Design review of the part built by this model. Coordinates are the model's own, in mm. Face numbers are marked on the shaded views. A direction names the side the tool comes from. Give positions to 0.01 mm unless a question says otherwise; leave off trailing zeros. Order: outer loops, then holes, each group sorted by start corner. A loop starts at its lowest first (then second) coordinate and runs counter-clockwise, first axis right, second up. Notation, with made-up numbers: (65.5, 33.5) -> (109.5, 33.5) arc R25 cw to (109.5, 45.5) -> close; hole circle Ø3 at (-8, 53). An arc over 180 degrees is marked (long way). One line per item, written item: value. Start each with the question number.
1) The part is to be moulded in two halves that separate along X. For the marked faces 1, 2 and 3, say which applies: released by +X, released by -X, zero draft, split by the parting line, or undercut.
2) Consider section C-C (y = 0). State the section outline as (x, z) points.
3) Wall thickness on line 1 along Y through (x, z) = (39, 2.5); line 2 along Y through (x, z) = (-21, 2.95); line 3 along Z through (x, y) = (-27, -4.5): over which ranges is each line inside the solid? List them lowest first. Write a range as from..to.
4) For pin 1 (7 mm diameter, centred on x = -21, y = 0, fed in from -Z), flat-tipped, find the tip position at first contact; note if it passes through.
5) Consider section A-A (z = 2). State the section outline as (x, y) points, plus the area to 3 significant figures.
6) Consider section B-B (x = -39). State the section outline as (y, z) points.
7) Tool access review of the marked faces 4 and 5: name each direction out of +Z, -Z, +X, -X, +Y, -Y from which nothing blocks a thin tool from reaching the whole face with its end or side.
8) Consider section D-D (x = -21). State the section outline as (y, z) points.
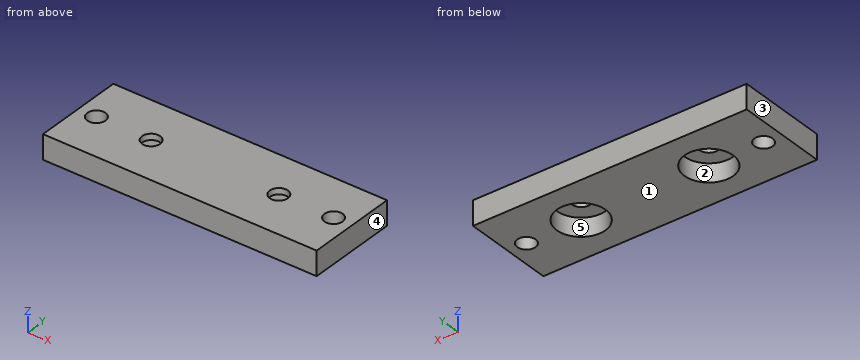
Autodesk Inventor part; units mm, degrees
ref_plane "YZ Plane" through (0, 0, 0) normal (1, 0, 0) x (0, 1, 0)
ref_plane "XZ Plane" through (0, 0, 0) normal (0, 1, 0) x (-1, 0, 0)
ref_plane "XY Plane" through (0, 0, 0) normal (0, 0, 1) x (1, 0, 0)
sketch "Sketch1" plane through (0, 0, 0) normal (0, 0, 1) x (1, 0, 0)
  circle A0 centre (-21, 0) radius 8
  circle A1 centre (21, 0) radius 8
  line L0 (-45, 15) -> (45, 15)
  line L1 (45, 15) -> (45, -15)
  line L2 (45, -15) -> (-45, -15)
  line L3 (-45, -15) -> (-45, 15)
  point P0 (0, 0)
  dimension "d0" = 16
  dimension "d1" = 16
  dimension "d2" = 42
  dimension "d3" = 21
  dimension "d4" = 15
  dimension "d5" = 30
  dimension "d6" = 16
  dimension "d7" = 16
extrude "Extrusion1" add sketch "Sketch1" along normal blind 8
sketch "Sketch2" plane through (0, 0, 8) normal (0, 0, 1) x (1, 0, 0)
  circle A0 centre (-21, 0) radius 8
  circle A1 centre (21, 0) radius 8
  point P0 (0, 0)
extrude "Extrusion2" add sketch "Sketch2" against normal blind 2
sketch "Sketch3" plane through (21, 0, 6) normal (0, 0, -1) x (-1, 0, 0)
  circle A0 centre (0, 0) radius 8
  circle A1 centre (42, 0) radius 8
  circle A2 centre (0, 0) radius 3
  circle A3 centre (42, 0) radius 3
  point P0 (21, 0)
  dimension "d12" = 6
  dimension "d13" = 6
extrude "Extrusion3" cut sketch "Sketch3" against normal through all contours A2 | A3
sketch "Sketch4" plane through (0, 0, 8) normal (0, 0, 1) x (1, 0, 0)
  circle A0 centre (-39, 0) radius 3
  circle A1 centre (39, 0) radius 3
  line L0 (-45, 15) -> (-45, -15)
  line L1 (45, 15) -> (45, -15)
  point P0 (0, 0)
  dimension "d16" = 6
  dimension "d17" = 6
  dimension "d18" = 6
  dimension "d19" = 6
extrude "Extrusion4" cut sketch "Sketch4" against normal through all
equation "\"d1\" = d0"
equation "\"d7\" = d6"
equation "\"d19\" = d18"
properties part number "bearing support"
Checked values:
1. face 1: zero draft
1. face 2: undercut
1. face 3: released by -X
2. outline: (-45, 0) -> (-42, 0) -> (-42, 8) -> (-45, 8) -> close; (-36, 0) -> (-29, 0) -> (-29, 6) -> (-24, 6) -> (-24, 8) -> (-36, 8) -> close; (-18, 6) -> (-13, 6) -> (-13, 0) -> (13, 0) -> (13, 6) -> (18, 6) -> (18, 8) -> (-18, 8) -> close; (24, 6) -> (29, 6) -> (29, 0) -> (36, 0) -> (36, 8) -> (24, 8) -> close; (42, 0) -> (45, 0) -> (45, 8) -> (42, 8) -> close
3. line 1: y = -15..-3, 3..15
3. line 2: y = -15..-8, 8..15
3. line 3: z = 6..8
4. pin 1: stops at z = 6
5. outline: (-45, -15) -> (45, -15) -> (45, 15) -> (-45, 15) -> close; hole circle Ø6 at (-39, 0); hole circle Ø16 at (-21, 0); hole circle Ø16 at (21, 0); hole circle Ø6 at (39, 0)
5. area: 2,240 mm^2
6. outline: (-15, 0) -> (-3, 0) -> (-3, 8) -> (-15, 8) -> close; (3, 0) -> (15, 0) -> (15, 8) -> (3, 8) -> close
7. face 4: +Z, -Z, +X, +Y, -Y
7. face 5: -Z
8. outline: (-15, 0) -> (-8, 0) -> (-8, 6) -> (-3, 6) -> (-3, 8) -> (-15, 8) -> close; (3, 6) -> (8, 6) -> (8, 0) -> (15, 0) -> (15, 8) -> (3, 8) -> close
